Input: part model. Units: mm. Frame: model coordinates. Face numbers are marked on the shaded views. Coordinates: 2 decimals unless noted, no trailing zeros. Write each loop counter-clockwise with the first axis right and the second up, starting at its lowest first coordinate (ties: lowest second). Pieces come first, ordered by that corner, then holes. Notation, with made-up numbers: (81, 29) -> (136, 29) arc R22 ccw to (136, 67) -> close; hole circle Ø2 at (58, -5). An arc over 180 degrees is marked (long way). Use one line per item in the form item = value. Start each with the question number.
(1) Cut plane B-B on y = 9. Return the cut outline in (x, z), plus the area to 3 significant figures.
(2) Pull-direction query (X, two-part tool) for the marked faces 1, 2 and 3; classes: released by +X, released by -X, zero draft, split by the parting line, or undercut.
(3) Ray query, line 1 along Y through (x, z) = (15, 4.5); line 2 along Z through (x, y) = (13.5, 1.5); line 3 along X through (y, z) = (7.5, 6.5). Return the intervals inside material, ascending.
(4) Cut plane A-A on x = 3. Return the cut outline in (y, z).
(5) First-contact query: pin 1 (2 mm diameter, centred on x = 33.5, y = 2.5, fed in from +Z); pin 2 (1.4 mm diameter, centred on y = 6.5, z = 7.5, fed in from -X); pin 3 (1.4 mm diameter, centred on x = 43.5, z = 6.5, fed in from -Y). Flat tips, straight axial feed; report the tip coordinate or a pass-through.
(6) Cut plane C-C on x = 25. Return the cut outline in (y, z).
(7) Cut plane D-D on y = 4.25. Return the cut outline in (x, z), plus the area to 3 significant figures.
```python
from build123d import *

# Parameters (mm, degrees)
SKETCH1_W           = 48
SKETCH1_H           = 12
BOSS_EXTRUDE1_DEPTH = 3
SKETCH2_W           = 35
SKETCH2_H           = 7
SKETCH2_W_2         = 1.3
SKETCH2_H_2         = 1.3
BOSS_EXTRUDE2_DEPTH = 8
SKETCH3_R           = 1
BOSS_EXTRUDE3_DEPTH = 8
FILLET1_R           = 1


with BuildPart() as part:
    # Sketch1 → Boss-Extrude1 (new body)
    with BuildSketch(Plane.XY):
        with Locations((24, 6)):
            Rectangle(SKETCH1_W, SKETCH1_H)
    extrude(amount=BOSS_EXTRUDE1_DEPTH)

    # Sketch2 → Boss-Extrude2 (add)
    with BuildSketch(Plane.XY.offset(3)):
        with Locations((30.5, 8.5)):
            Rectangle(SKETCH2_W, SKETCH2_H)
        with Locations((17.25, 10.35)):
            Rectangle(SKETCH2_W_2, SKETCH2_H_2, mode=Mode.SUBTRACT)
        with Locations((14.65, 10.35)):
            Rectangle(SKETCH2_W_2, SKETCH2_H_2, mode=Mode.SUBTRACT)
        with Locations((14.65, 6.65)):
            Rectangle(SKETCH2_W_2, SKETCH2_H_2, mode=Mode.SUBTRACT)
        with Locations((17.25, 6.65)):
            Rectangle(SKETCH2_W_2, SKETCH2_H_2, mode=Mode.SUBTRACT)
        with Locations((19.85, 10.35)):
            Rectangle(SKETCH2_W_2, SKETCH2_H_2, mode=Mode.SUBTRACT)
        with Locations((19.85, 6.65)):
            Rectangle(SKETCH2_W_2, SKETCH2_H_2, mode=Mode.SUBTRACT)
        with Locations((22.45, 10.35)):
            Rectangle(SKETCH2_W_2, SKETCH2_H_2, mode=Mode.SUBTRACT)
        with Locations((22.45, 6.65)):
            Rectangle(SKETCH2_W_2, SKETCH2_H_2, mode=Mode.SUBTRACT)
        with Locations((25.05, 10.35)):
            Rectangle(SKETCH2_W_2, SKETCH2_H_2, mode=Mode.SUBTRACT)
        with Locations((25.05, 6.65)):
            Rectangle(SKETCH2_W_2, SKETCH2_H_2, mode=Mode.SUBTRACT)
        with Locations((27.65, 10.35)):
            Rectangle(SKETCH2_W_2, SKETCH2_H_2, mode=Mode.SUBTRACT)
        with Locations((27.65, 6.65)):
            Rectangle(SKETCH2_W_2, SKETCH2_H_2, mode=Mode.SUBTRACT)
        with Locations((30.25, 10.35)):
            Rectangle(SKETCH2_W_2, SKETCH2_H_2, mode=Mode.SUBTRACT)
        with Locations((30.25, 6.65)):
            Rectangle(SKETCH2_W_2, SKETCH2_H_2, mode=Mode.SUBTRACT)
        with Locations((32.85, 10.35)):
            Rectangle(SKETCH2_W_2, SKETCH2_H_2, mode=Mode.SUBTRACT)
        with Locations((32.85, 6.65)):
            Rectangle(SKETCH2_W_2, SKETCH2_H_2, mode=Mode.SUBTRACT)
        with Locations((35.45, 10.35)):
            Rectangle(SKETCH2_W_2, SKETCH2_H_2, mode=Mode.SUBTRACT)
        with Locations((35.45, 6.65)):
            Rectangle(SKETCH2_W_2, SKETCH2_H_2, mode=Mode.SUBTRACT)
        with Locations((38.05, 10.35)):
            Rectangle(SKETCH2_W_2, SKETCH2_H_2, mode=Mode.SUBTRACT)
        with Locations((38.05, 6.65)):
            Rectangle(SKETCH2_W_2, SKETCH2_H_2, mode=Mode.SUBTRACT)
        with Locations((40.65, 10.35)):
            Rectangle(SKETCH2_W_2, SKETCH2_H_2, mode=Mode.SUBTRACT)
        with Locations((40.65, 6.65)):
            Rectangle(SKETCH2_W_2, SKETCH2_H_2, mode=Mode.SUBTRACT)
        with Locations((43.25, 10.35)):
            Rectangle(SKETCH2_W_2, SKETCH2_H_2, mode=Mode.SUBTRACT)
        with Locations((43.25, 6.65)):
            Rectangle(SKETCH2_W_2, SKETCH2_H_2, mode=Mode.SUBTRACT)
        with Locations((45.85, 10.35)):
            Rectangle(SKETCH2_W_2, SKETCH2_H_2, mode=Mode.SUBTRACT)
        with Locations((45.85, 6.65)):
            Rectangle(SKETCH2_W_2, SKETCH2_H_2, mode=Mode.SUBTRACT)
    extrude(amount=BOSS_EXTRUDE2_DEPTH)

    # Sketch3 → Boss-Extrude3 (add)
    with BuildSketch(Plane.XY.offset(3)):
        with Locations(Location((3, 9, 0), (0, 0, 180))):
            Circle(SKETCH3_R)
        with Locations(Location((3, 6, 0), (0, 0, 180))):
            Circle(SKETCH3_R)
        with Locations(Location((6, 9, 0), (0, 0, 180))):
            Circle(SKETCH3_R)
        with Locations(Location((6, 6, 0), (0, 0, 180))):
            Circle(SKETCH3_R)
    extrude(amount=BOSS_EXTRUDE3_DEPTH)

    # Fillet1
    fillet1_edges = [part.edges().sort_by_distance(p)[0] for p in [
        (4, 9, 11),
        (4, 6, 11),
        (7, 9, 11),
        (7, 6, 11),
    ]]
    fillet(fillet1_edges, radius=FILLET1_R)


solid = part.part
```
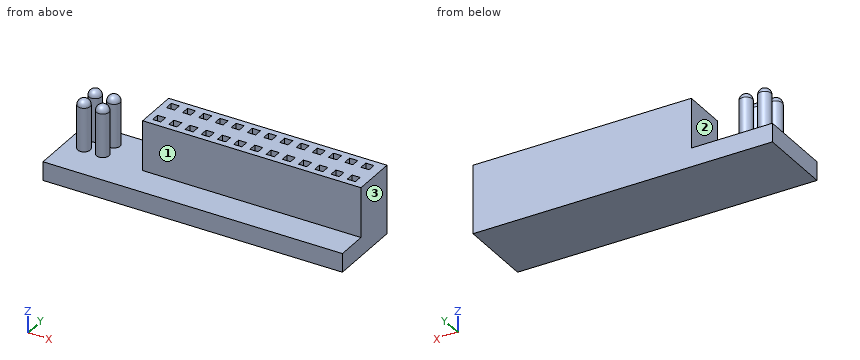
Values:
q1.outline = (0, 0) -> (48, 0) -> (48, 11) -> (13, 11) -> (13, 3) -> (7, 3) -> (7, 10) arc R1 ccw to (5, 10) -> (5, 3) -> (4, 3) -> (4, 10) arc R1 ccw to (2, 10) -> (2, 3) -> (0, 3) -> close
q1.area = 455 mm2
q2.face_1 = zero draft
q2.face_2 = undercut
q2.face_3 = released by +X
q3.line_1 = 5 to 6, 7.3 to 9.7, 11 to 12
q3.line_2 = 0 to 3
q3.line_3 = 13 to 48
q4.outline = (0, 0) -> (12, 0) -> (12, 3) -> (10, 3) -> (10, 10) arc R1 ccw to (8, 10) -> (8, 3) -> (7, 3) -> (7, 10) arc R1 ccw to (5, 10) -> (5, 3) -> (0, 3) -> close
q5.pin_1 = 3
q5.pin_2 = 2
q5.pin_3 = 5
q6.outline = (0, 0) -> (12, 0) -> (12, 11) -> (11, 11) -> (11, 3) -> (9.7, 3) -> (9.7, 11) -> (7.3, 11) -> (7.3, 3) -> (6, 3) -> (6, 11) -> (5, 11) -> (5, 3) -> (0, 3) -> close
q7.outline = (0, 0) -> (48, 0) -> (48, 3) -> (0, 3) -> close
q7.area = 144 mm2
